```python
from build123d import *

# Parameters (mm, degrees)
BOSS_EXTRUDE1_DEPTH      = 6.35
BOSS_EXTRUDE1_DEPTH_BACK = 3.302
SKETCH3_R                = 4.826
SKETCH4_R                = 1.651
CUT_EXTRUDE1_DEPTH       = 24.759524406
CUT_EXTRUDE2_DEPTH       = 33.378773911
FILLET1_R                = 2.4765


with BuildPart() as part:
    # Sketch3 → Boss-Extrude1 (new, two sides: drawn at the far end of the back side and taken through both)
    with BuildSketch(Plane.XY.offset(-BOSS_EXTRUDE1_DEPTH_BACK)):
        with BuildLine():
            Line((-12.7, 0), (12.7, 0))
            Line((12.7, 0), (12.7, 3.048))
            Line((12.7, 3.048), (7.083102209, 14.615409702))
            ThreePointArc((7.083102209, 14.615409702), (0, 19.05), (-7.083102209, 14.615409702))
            Line((-7.083102209, 14.615409702), (-12.7, 3.048))
            Line((-12.7, 3.048), (-12.7, 0))
        make_face()
        with Locations((0, 11.176)):
            Circle(SKETCH3_R, mode=Mode.SUBTRACT)
    extrude(amount=BOSS_EXTRUDE1_DEPTH + BOSS_EXTRUDE1_DEPTH_BACK)

    # Sketch4 → Cut-Extrude1 (cut, through all)
    with BuildSketch(Plane(origin=(0, 0, 0), x_dir=(1, 0, 0), z_dir=(0, 1, 0))):
        with Locations((9.652, 0)):
            Circle(SKETCH4_R)
        with Locations(Location((-9.652, 0, 0), (0, 0, 180))):
            Circle(SKETCH4_R)
    extrude(amount=CUT_EXTRUDE1_DEPTH, mode=Mode.SUBTRACT)

    # Sketch5 → Cut-Extrude2 (cut, through all)
    with BuildSketch(Plane.ZY.offset(12.7)):
        with BuildLine():
            Line((-3.302, 19.05), (4.826, 19.05))
            Line((4.826, 19.05), (4.826, 2.286))
            ThreePointArc((4.826, 2.286), (4.602815367, 1.747184633), (4.064, 1.524))
            Line((4.064, 1.524), (-3.302, 1.524))
            Line((-3.302, 1.524), (-3.302, 19.05))
        make_face()
        with BuildLine():
            Line((4.064, 0), (6.35, 0))
            Line((6.35, 0), (6.35, 2.286))
            ThreePointArc((6.35, 2.286), (5.680446102, 0.669553898), (4.064, 0))
        make_face()
    extrude(amount=-CUT_EXTRUDE2_DEPTH, mode=Mode.SUBTRACT)

    # Fillet1
    fillet1_edges = [part.edges().sort_by_distance(p)[0] for p in [
        (12.7, 0.762, -3.302),
        (-12.7, 0.762, -3.302),
    ]]
    fillet(fillet1_edges, radius=FILLET1_R)


solid = part.part
```
Could you check a few things on this model? Use its own coordinates, in mm. A direction names the side the tool comes from. Give positions to 0.01 mm unless a question says otherwise; leave off trailing zeros. Loops run counter-clockwise (first coordinate to the right, second up) from the corner with the lowest first, then second, coordinate; pieces in that order, holes last. Notation, with made-up numbers: (57, 36.5) - (68, 36.5) arc R22 ccw to (68, 45.5) - close; hole circle Ø8 at (-29, 44). An arc over 180 degrees is marked (long way). Use one line per item in the form item = value.
1. I want a section at B-B (x = 0). Please give me the cut outline in (y, z), and give its area (3 significant figures).
Response values:
outline = (0, -3.3) - (1.52, -3.3) - (1.52, 4.06) arc R0.76 cw to (2.29, 4.83) - (6.35, 4.83) - (6.35, 6.35) - (2.29, 6.35) arc R2.29 ccw to (0, 4.06) - close; (16, 4.83) - (19.05, 4.83) - (19.05, 6.35) - (16, 6.35) - close
area = 25.7 mm²
2. On a 3-axis mill with a long thin cutter (end or side, diameter ignored), from which of +Z, -Z, +X, -X, +Y, -Y can I reach the whole of each face in a straight line? I mean faces 1 (the face through (8.34, 0.75, 1)), 2 (the face through (0, 1.524, 0)). Say none if no direction works.
Response values:
face_1 = +Y, -Y
face_2 = -Z, +X, -X, +Y
3. Thinking about a two-plate mould opening in X: for faces 3 (the face through (-12.7, 1, 4)), 4 (the face through (-11.227, 0.751, 0.496)), 5 (the face through (0, 0, 0)), which applies, released by +X, released by -X, zero draft, split by the parting line, or undercut?
Response values:
face_3 = released by -X
face_4 = undercut
face_5 = zero draft
4. I want a section at D-D (x = -9.25). Please give me the cut outline in (y, z), and give its area (3 significant figures).
Response values:
outline = (0, -3.3) - (1.52, -3.3) - (1.52, -1.6) - (0, -1.6) - close; (0, 1.6) - (1.52, 1.6) - (1.52, 4.06) arc R0.76 cw to (2.29, 4.83) - (10.15, 4.83) - (10.15, 6.35) - (2.29, 6.35) arc R2.29 ccw to (0, 4.06) - close
area = 22.0 mm²
5. I want a section at A-A (z = 0). Please give me the cut outline in (x, y), and give its area (3 significant figures).
Response values:
outline = (-12.7, 0) - (-11.3, 0) - (-11.3, 1.52) - (-12.7, 1.52) - close; (-8, 0) - (8, 0) - (8, 1.52) - (-8, 1.52) - close; (11.3, 0) - (12.7, 0) - (12.7, 1.52) - (11.3, 1.52) - close
area = 28.6 mm²
6. I'm going to push flat-ended pins straight in: pin 1 Ø2 at (x, y) = (-8.5, 17) entering from -Z; pin 2 Ø5.5 at (x, z) = (-9.652, 0) entering from +Y; pin 3 Ø8 at (x, y) = (4.5, 8.5) entering from -Z; pin 4 Ø5 at (y, z) = (7, 3) entering from +X. Where does each tip first touch, or does it pass through?
Response values:
pin_1 = through
pin_2 = 1.52
pin_3 = 4.83
pin_4 = 11.61
7. I need wall thicknesses on probe 1 along X at (y, z) = (0.75, 0); probe 2 along Z at (x, y) = (-7, 8.5); probe 3 along Y at (x, z) = (2, 4). Which ranges of each line are inside material? Lowest first, please.
Response values:
probe_1 = -12.7 to -11.3, -8 to 8, 11.3 to 12.7
probe_2 = 4.83 to 6.35
probe_3 = 0 to 1.52
8. I want a section at C-C (y = 7.75). Please give me the cut outline in (x, z), and give its area (3 significant figures).
Response values:
outline = (-10.42, 4.83) - (-3.4, 4.83) - (-3.4, 6.35) - (-10.42, 6.35) - close; (3.4, 4.83) - (10.42, 4.83) - (10.42, 6.35) - (3.4, 6.35) - close
area = 21.4 mm²
